Verification items for this drawing (mm, ordinates from the low corner). Round coordinates to 2 decimals unless told otherwise and drop trailing zeros. Order: outer loops, then holes, each group sorted by start corner. A loop starts at its lowest first (then second) coordinate and runs counter-clockwise, first axis right, second up. Notation, with made-up numbers: M -20.75,-30 L -4.75,-30 A29 ccw -4.75,1 Z; hole C -15,66.5 d5. An arc over 180 degrees is marked long. One line per item, written item: value. Start each with the question number.
(1) Cross-section at B-B, the plane x = 51.5. Enter the section's corners in (y, z).
(2) Cross-section at A-A, the plane y = 2.3. Enter the section's corners in (x, z), and give its area (3 significant figures).
(3) Thickness scan on L1, parallel to X at y = 3.5, z = 8.25; L2, parallel to Y at x = 42, z = 2.25; L3, parallel to Z at x = 60, y = 3.4. Record the ranges inside material, lowest first.
(4) Depth check by flat-ended pin: pin 1 Ø1.2 at (y, z) = (1.5, 6.5) entering from -X; pin 2 Ø6 at (x, z) = (71.5, 8) entering from -Y; pin 3 Ø2 at (x, y) = (56, 1.5) entering from -Z. Enter the tip coordinate at first touch or a pass-through.
(5) Cross-section at D-D, the plane x = 40.5. Enter the section's corners in (y, z), and give its area (3 significant figures).
(6) Cross-section at C-C, the plane z = 4.25. Enter the section's corners in (x, y), and give its area (3 significant figures).
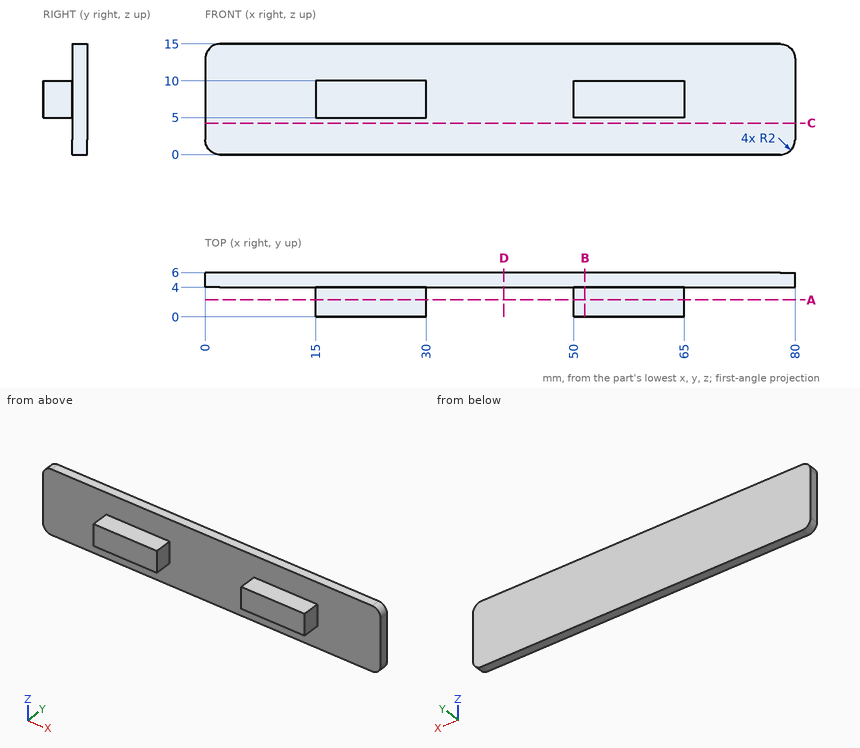
Values found:
1. outline: M 0,5 L 4,5 L 4,0 L 6,0 L 6,15 L 4,15 L 4,10 L 0,10 Z
2. outline: M 15,5 L 30,5 L 30,10 L 15,10 Z; M 50,5 L 65,5 L 65,10 L 50,10 Z
2. area: 150 mm^2
3. L1: 15 to 30, 50 to 65
3. L2: 4 to 6
3. L3: 5 to 10
4. pin 1: x = 15
4. pin 2: y = 4
4. pin 3: z = 5
5. outline: M 4,0 L 6,0 L 6,15 L 4,15 Z
5. area: 30.0 mm^2
6. outline: M 0,4 L 80,4 L 80,6 L 0,6 Z
6. area: 160 mm^2
